from build123d import *

# Parameters (mm, degrees)
SZKIC1_W                    = 20
SZKIC1_H                    = 14
SZKIC1_R                    = 1.5
DODANIE_WYCI_GNI_CIE1_DEPTH = 3
ZAOKR_GLENIE5_R             = 2
ZAOKR_GLENIE6_R             = 5


with BuildPart() as part:
    # Szkic1 → Dodanie-wyciągnięcie1 (new body)
    # profile 1 of 2: a face of its own
    with BuildSketch(Plane.XY):
        Rectangle(SZKIC1_W, SZKIC1_H)
        with Locations((-6, -4)):
            Circle(SZKIC1_R, mode=Mode.SUBTRACT)
        with Locations((6, -4)):
            Circle(SZKIC1_R, mode=Mode.SUBTRACT)
        with Locations((6, 4)):
            Circle(SZKIC1_R, mode=Mode.SUBTRACT)
        with Locations((-6, 4)):
            Circle(SZKIC1_R, mode=Mode.SUBTRACT)
    # profile 2 of 2: a face of its own
    with BuildSketch(Plane.XY):
        with BuildLine():
            Line((10, -4), (10, -7))
            Line((10, -7), (47.5, -7))
            Line((47.5, -7), (47.5, -3.5))
            ThreePointArc((47.5, -3.5), (44.249121219, -0.510508432), (41.541960108, -4))
            Line((41.541960108, -4), (10, -4))
        make_face()
        with Locations((44.5, -3.5)):
            Circle(SZKIC1_R, mode=Mode.SUBTRACT)
    extrude(amount=DODANIE_WYCI_GNI_CIE1_DEPTH)

    # Zaokrąglenie5
    zaokr_glenie5_edges = [part.edges().sort_by_distance(p)[0] for p in [
        (-10, 7, 1.5),
        (10, 7, 1.5),
        (47.5, -7, 1.5),
        (-10, -7, 1.5),
    ]]
    fillet(zaokr_glenie5_edges, radius=ZAOKR_GLENIE5_R)

    # Zaokrąglenie6
    zaokr_glenie6_edges = [part.edges().sort_by_distance(p)[0] for p in [
        (10, -4, 1.5),
        (41.541960108, -4, 1.5),
    ]]
    fillet(zaokr_glenie6_edges, radius=ZAOKR_GLENIE6_R)


solid = part.part
Can you work these out from the model? Positions are in its coordinate system, mm. A direction names the side the tool comes from. Give positions to 0.01 mm unless a question says otherwise; leave off trailing zeros. Order: outer loops, then holes, each group sorted by start corner. A loop starts at its lowest first (then second) coordinate and runs counter-clockwise, first axis right, second up. Notation, with made-up numbers: M -6,-3 L 40,-3 A24 cw 40,26 Z; hole C -13,18.5 d7. An arc over 180 degrees is marked long. One line per question, with ' | ' between items.
Item 1: I'm going to push flat-ended pins straight in: pin 1 Ø1.8 at (x, y) = (-6, 4) entering from +Z; pin 2 Ø1.5 at (y, z) = (3.5, 1.5) entering from +X; pin 3 Ø0.9 at (x, z) = (30.5, 1.5) entering from +Y. Where does each tip first touch, or does it pass through?
Answer block:
pin 1: passes through | pin 2: stops at x = 10 | pin 3: stops at y = -4
Item 2: For faces 1 (the face through (27, -4, 1)), 2 (the face through (0, 7, 1)), which set-ups out of +Z, -Z, +X, -X, +Y, -Y let a thin tool reach every point of the face, with its end or its side?
Answer block:
face 1: +Z, -Z, +Y | face 2: +Z, -Z, +X, -X, +Y
Item 3: Suppose I cut it at B-B, the plane y = 4. Write out the boundary of the cut face in (x, z).
Answer block:
outline: M -10,0 L -7.5,0 L -7.5,3 L -10,3 Z; M -4.5,0 L 4.5,0 L 4.5,3 L -4.5,3 Z; M 7.5,0 L 10,0 L 10,3 L 7.5,3 Z
Item 4: Suppose I cut it at A-A, the plane z = 0.65. Write out the boundary of the cut face in (x, y).
Answer block:
outline: M -10,-5 A2 ccw -8,-7 L 45.5,-7 A2 ccw 47.5,-5 L 47.5,-3.5 A3 ccw 42.02,-1.81 A5 cw 37.89,-4 L 15,-4 A5 cw 10,1 L 10,5 A2 ccw 8,7 L -8,7 A2 ccw -10,5 Z; hole C -6,-4 d3; hole C -6,4 d3; hole C 6,-4 d3; hole C 6,4 d3; hole C 44.5,-3.5 d3
Item 5: Please list where these lines run through material, in increasing order: L1, parallel to Y at x = 6, z = 2.45; L2, parallel to X at y = 3.25, z = 0.3; L3, parallel to Y at x = 5.5, z = 2.65.
Answer block:
L1: y = -7 to -5.5, -2.5 to 2.5, 5.5 to 7 | L2: x = -10 to -7.3, -4.7 to 4.7, 7.3 to 10 | L3: y = -7 to -5.41, -2.59 to 2.59, 5.41 to 7
Item 6: Suppose I cut it at D-D, the plane x = 44.5. Write out the boundary of the cut face in (y, z), then the cut area to 3 significant figures.
Answer block:
outline: M -7,0 L -5,0 L -5,3 L -7,3 Z; M -2,0 L -0.5,0 L -0.5,3 L -2,3 Z | area: 10.5 mm2
Item 7: Suppose I cut it at C-C, the plane x = 6. Write out the boundary of the cut face in (y, z), then the cut area to 3 significant figures.
Answer block:
outline: M -7,0 L -5.5,0 L -5.5,3 L -7,3 Z; M -2.5,0 L 2.5,0 L 2.5,3 L -2.5,3 Z; M 5.5,0 L 7,0 L 7,3 L 5.5,3 Z | area: 24.0 mm2
Item 8: We'd pull the mould along Y, two halves only. Please class faces 3 (the face through (40.194, -3.435, 1.521)), 4 (the face through (46.93, -6.4, 1.52)), 5 (the face through (12, -5, 0)), 6 (the face through (43, -3.43, 1.48)): released by +Y, released by -Y, zero draft, split by the parting line, or undercut.
Answer block:
face 3: released by +Y | face 4: released by -Y | face 5: zero draft | face 6: undercut
